```python
from build123d import *

# Parameters (mm, degrees)
F0_R     = 7.99973
F1_DEPTH = 6.35
F2_R     = 12.7
F3_DEPTH = 1.5875
F6_D     = 2.7051
F6_DEPTH = 19.05
F6_START = 2.9673452
F6_TIP   = 0.8126940303


with BuildPart() as f1:
    # F0 (on Top) → F1 (new body)
    with BuildSketch(Plane.XY):
        with BuildLine():
            ThreePointArc((3.1682020813, 24.0648839888), (0, 21.0975389242), (-3.1682020813, 24.0648839888))
            ThreePointArc((-3.1682020813, 24.0648839888), (-6.2821953466, 23.4454722164), (-9.2886985077, 22.4249019141))
            ThreePointArc((-9.2886985077, 22.4249019141), (-10.5487694621, 18.2710046656), (-14.7761854811, 19.2566998328))
            ThreePointArc((-14.7761854811, 19.2566998328), (-17.1632768699, 17.1632768699), (-19.2566998328, 14.7761854811))
            ThreePointArc((-19.2566998328, 14.7761854811), (-18.2710046656, 10.5487694621), (-22.4249019141, 9.2886985077))
            ThreePointArc((-22.4249019141, 9.2886985077), (-23.4454722164, 6.2821953466), (-24.0648839888, 3.1682020813))
            ThreePointArc((-24.0648839888, 3.1682020813), (-21.0975389242, 0), (-24.0648839888, -3.1682020813))
            ThreePointArc((-24.0648839888, -3.1682020813), (-23.4454722164, -6.2821953466), (-22.4249019141, -9.2886985077))
            ThreePointArc((-22.4249019141, -9.2886985077), (-18.2710046656, -10.5487694621), (-19.2566998328, -14.7761854811))
            ThreePointArc((-19.2566998328, -14.7761854811), (-17.1632768699, -17.1632768699), (-14.7761854811, -19.2566998328))
            ThreePointArc((-14.7761854811, -19.2566998328), (-10.5487694621, -18.2710046656), (-9.2886985077, -22.4249019141))
            ThreePointArc((-9.2886985077, -22.4249019141), (-6.2821953466, -23.4454722164), (-3.1682020813, -24.0648839888))
            ThreePointArc((-3.1682020813, -24.0648839888), (0, -21.0975389242), (3.1682020813, -24.0648839888))
            ThreePointArc((3.1682020813, -24.0648839888), (6.2821953466, -23.4454722164), (9.2886985077, -22.4249019141))
            ThreePointArc((9.2886985077, -22.4249019141), (10.5487694621, -18.2710046656), (14.7761854811, -19.2566998328))
            ThreePointArc((14.7761854811, -19.2566998328), (17.1632768699, -17.1632768699), (19.2566998328, -14.7761854811))
            ThreePointArc((19.2566998328, -14.7761854811), (18.2710046656, -10.5487694621), (22.4249019141, -9.2886985077))
            ThreePointArc((22.4249019141, -9.2886985077), (23.4454722164, -6.2821953466), (24.0648839888, -3.1682020813))
            ThreePointArc((24.0648839888, -3.1682020813), (21.0975389242, 0), (24.0648839888, 3.1682020813))
            ThreePointArc((24.0648839888, 3.1682020813), (23.4454722164, 6.2821953466), (22.4249019141, 9.2886985077))
            ThreePointArc((22.4249019141, 9.2886985077), (18.2710046656, 10.5487694621), (19.2566998328, 14.7761854811))
            ThreePointArc((19.2566998328, 14.7761854811), (17.1632768699, 17.1632768699), (14.7761854811, 19.2566998328))
            ThreePointArc((14.7761854811, 19.2566998328), (10.5487694621, 18.2710046656), (9.2886985077, 22.4249019141))
            ThreePointArc((9.2886985077, 22.4249019141), (6.2821953466, 23.4454722164), (3.1682020813, 24.0648839888))
        make_face()
        Circle(F0_R, mode=Mode.SUBTRACT)
    extrude(amount=F1_DEPTH)

    # F2 (on face) → F3 (cut)
    with BuildSketch(Plane.XY.offset(6.35)):
        Circle(F2_R)
    extrude(amount=-F3_DEPTH, mode=Mode.SUBTRACT)

    # F6
    # its depths count from where the whole tool has entered the part; down to there all is cleared
    with Locations(Plane(origin=(0, 24.0648839888, 0), x_dir=(1, 0, 0), z_dir=(0, 1, 0)).offset(-F6_START)):
        with Locations((0, -2.38125)):
            Hole(F6_D / 2, depth=F6_DEPTH)
            with Locations((0, 0, -(F6_DEPTH + F6_TIP / 2))):  # 118° drill point
                Cone(0, F6_D / 2, F6_TIP, mode=Mode.SUBTRACT)


solid = f1.part
```
Geometry check sheet. Reference: the model listing, model coordinates, mm. A direction names the side the tool comes from. Coordinates: 2 decimals unless noted, no trailing zeros. Order: outer loops, then holes, each group sorted by start corner. A loop starts at its lowest first (then second) coordinate and runs counter-clockwise, first axis right, second up.
Item 1: Section check D-D (y = -5.5). Enter the section's corners in (x, z).
Item 2: Section check C-C (y = 12). Enter the section's corners in (x, z).
Item 3: Tool access check on faces 1 (the cylindrical face through (-18.3, -10.5, 3.1)), 2 (the cylindrical face through (0.3, 14.5, 3.7)). Record the directions out of +Z, -Z, +X, -X, +Y, -Y that give a thin tool (end or side, any length) a straight path to the whole face; none if there is none.
Item 4: Mould release check, pull along X, two halves, no side actions. Record for faces 3 (the cylindrical face through (-0.1, -21.1, 3.1)), 4 (the flat face through (10, -10, 6.35)), 5 (the cylindrical face through (21.1, -0.1, 3.1)): released by +X, released by -X, zero draft, split by the parting line, or undercut.
Item 5: Scan lines: line 1 along Y through (x, z) = (0, 5.7); line 2 along X through (y, z) = (19, 0.5); line 3 along Z through (x, y) = (0, 13). Record each from-to range of solid material in increasing order.
Item 6: Section check A-A (x = 0). Enter the section's corners in (y, z), plus the area to 3 significant figures.
Item 7: Depth check by flat-ended pin: pin 1 (2 mm diameter, centred on x = -18.5, y = 13.5, fed in from +Z); pin 2 (12.5 mm diameter, centred on x = -2.5, y = 0, fed in from +Z); pin 3 (14.5 mm diameter, centred on x = 0, y = 0, fed in from +Z); pin 4 (2 mm diameter, centred on y = 8, z = 1, fed in from -X). Enter the tip coordinate at first touch or a pass-through.
Item 8: Section check B-B (y = 0). Enter the section's corners in (x, z).
Check sheet entries:
1. outline: (-23.64, 0) - (-5.81, 0) - (-5.81, 4.76) - (-11.45, 4.76) - (-11.45, 6.35) - (-23.64, 6.35) - close; (5.81, 0) - (23.64, 0) - (23.64, 6.35) - (11.45, 6.35) - (11.45, 4.76) - (5.81, 4.76) - close
2. outline: (-17.85, 0) - (17.85, 0) - (17.85, 6.35) - (4.16, 6.35) - (4.16, 4.76) - (-4.16, 4.76) - (-4.16, 6.35) - (-17.85, 6.35) - close; hole circle Ø2.71 at (0, 2.38)
3. face 1: +Z, -Z
3. face 2: +Y
4. face 3: undercut
4. face 4: zero draft
4. face 5: released by +X
5. line 1: y = -21.1 to -12.7, 12.7 to 21.1
5. line 2: x = -15.1 to -14.59, -9.69 to 9.69, 14.59 to 15.1
5. line 3: z = 0 to 1.03, 3.73 to 6.35
6. outline: (-21.1, 0) - (-8, 0) - (-8, 4.76) - (-12.7, 4.76) - (-12.7, 6.35) - (-21.1, 6.35) - close; (8, 0) - (21.1, 0) - (21.1, 1.03) - (8, 1.03) - close; (8, 3.73) - (21.1, 3.73) - (21.1, 6.35) - (12.7, 6.35) - (12.7, 4.76) - (8, 4.76) - close
6. area: 116 mm2
7. pin 1: stops at z = 6.35
7. pin 2: stops at z = 4.76
7. pin 3: passes through
7. pin 4: stops at x = -23.24
8. outline: (-21.1, 0) - (-8, 0) - (-8, 4.76) - (-12.7, 4.76) - (-12.7, 6.35) - (-21.1, 6.35) - close; (8, 0) - (21.1, 0) - (21.1, 6.35) - (12.7, 6.35) - (12.7, 4.76) - (8, 4.76) - close
